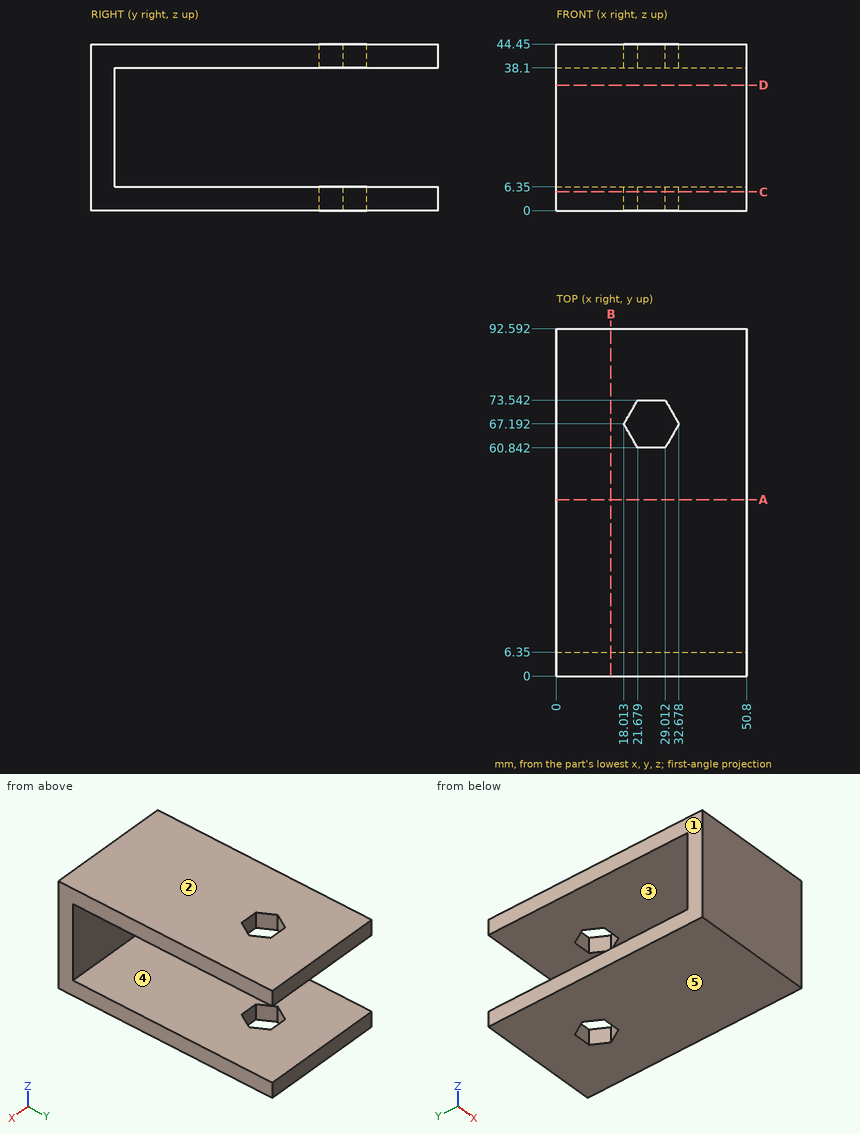
Check sheet for the drawn part. Datum: minimum x, y, z corner. Units: mm. A direction names the side the tool comes from. Coordinates: 2 decimals unless noted, no trailing zeros. Loops run counter-clockwise (first coordinate to the right, second up) from the corner with the lowest first, then second, coordinate; pieces in that order, holes last. Notation, with made-up numbers: M 51,-2 L 92,-2 A22 cw 92,14 Z; hole C 83,51.25 d11. An arc over 180 degrees is marked long. Answer as a JSON object with one key per item and string values.
1. Sectioned sample at C-C on z = 5. Record the cut outline in (x, y), and give its area (3 significant figures).
Outcome:
{"outline": "M 0,0 L 50.8,0 L 50.8,92.59 L 0,92.59 Z; hole M 18.01,67.19 L 21.68,60.84 L 29.01,60.84 L 32.68,67.19 L 29.01,73.54 L 21.68,73.54 Z", "area": "4,560 mm²"}
2. Scan lines: L1, parallel to Z at x = 5.5, y = 32; L2, parallel to Y at x = 26, z = 31.5; L3, parallel to Y at x = 26.5, z = 39. Record each from-to range of solid material in increasing order. Write a range as from..to.
Outcome:
{"L1": "0..6.35, 38.1..44.45", "L2": "0..6.35", "L3": "0..60.84, 73.54..92.59"}
3. Access from +Z, -Z, +X, -X, +Y, -Y to the whole of each face (thin tool, end or side, straight path). Record for the marked faces 4 and 5.
Outcome:
{"face 4": "+X, -X, +Y", "face 5": "-Z, +X, -X, +Y, -Y"}
4. Sectioned sample at A-A on y = 47. Record the cut outline in (x, z), and give its area (3 significant figures).
Outcome:
{"outline": "M 0,0 L 50.8,0 L 50.8,6.35 L 0,6.35 Z; M 0,38.1 L 50.8,38.1 L 50.8,44.45 L 0,44.45 Z", "area": "645 mm²"}
5. Sectioned sample at B-B on x = 14.5. Record the cut outline in (y, z), and give its area (3 significant figures).
Outcome:
{"outline": "M 0,0 L 92.59,0 L 92.59,6.35 L 6.35,6.35 L 6.35,38.1 L 92.59,38.1 L 92.59,44.45 L 0,44.45 Z", "area": "1,380 mm²"}
6. Sectioned sample at D-D on z = 33.5. Record the cut outline in (x, y).
Outcome:
{"outline": "M 0,0 L 50.8,0 L 50.8,6.35 L 0,6.35 Z"}
7. Release check for a two-part mould opening along Z. For the marked faces 1, 2 and 3 record: pulls with the +Z half, pulls with the -Z half, needs draft (parallel to the pull), parting line crosses it, or undercut.
Outcome:
{"face 1": "needs draft", "face 2": "pulls with the +Z half", "face 3": "undercut"}
8. Depth check by flat-ended pin: P1, Ø4, axis at x = 27, z = 33, coming from the +Y side. Enter the tip coordinate at first touch or a pass-through.
Outcome:
{"P1": "y = 6.35"}
